from build123d import *

# Parameters (mm, degrees)
F0_R           = 1.6
F1_DEPTH       = 4
F2_W           = 15.6
F2_H           = 14.6
F3_DEPTH       = 5.4
F4_W           = 15.6
F4_H           = 3
F5_DEPTH       = 0.4
F8_D           = 2
F8_DEPTH       = 5
F8_TIP         = 0.600860619
F8_ON_F7_D     = 2
F8_ON_F7_DEPTH = 5
F8_ON_F7_TIP   = 0.600860619
F10_DEPTH      = 25
F12_DEPTH      = 3


with BuildPart() as f1:
    # F0 (on Front) → F1 (new body)
    with BuildSketch(Plane.XZ):
        with BuildLine():
            Line((-7.8, 6.3143593539), (-7.8, 0))
            Line((-7.8, 0), (7.8, 0))
            Line((7.8, 0), (7.8, 6.3143593539))
            ThreePointArc((7.8, 6.3143593539), (5.4, 7.7), (7.8, 9.0856406461))
            Line((7.8, 9.0856406461), (7.8, 20.2))
            Line((7.8, 20.2), (-7.8, 20.2))
            Line((-7.8, 20.2), (-7.8, 9.0856406461))
            ThreePointArc((-7.8, 9.0856406461), (-6.2, 9.0856406461), (-5.4, 7.7))
            ThreePointArc((-5.4, 7.7), (-6.2, 6.3143593539), (-7.8, 6.3143593539))
        make_face()
        with Locations((0, 17.7)):
            Circle(F0_R, mode=Mode.SUBTRACT)
    extrude(amount=F1_DEPTH)

    # F2 (on Front) → F3 (join)
    with BuildSketch(Plane.XZ):
        with Locations((0, -2.7)):
            Rectangle(F2_W, F2_H)
    extrude(amount=-F3_DEPTH)

    # F4 (on face) → F5 (join)
    with BuildSketch(Plane.XZ):
        with Locations((0, -8.5)):
            Rectangle(F4_W, F4_H)
    extrude(amount=F5_DEPTH)

    # F8
    with Locations(Plane.YZ.offset(7.8)):
        with Locations((2.9, -5)):
            Hole(F8_D / 2, depth=F8_DEPTH)
            with Locations((0, 0, -(F8_DEPTH + F8_TIP / 2))):  # 118° drill point
                Cone(0, F8_D / 2, F8_TIP, mode=Mode.SUBTRACT)

    # F8 on F7
    with Locations(Plane(origin=(-7.8, 0, 0), x_dir=(0, -1, 0), z_dir=(-1, 0, 0))):
        with Locations((-2.9, -5)):
            Hole(F8_ON_F7_D / 2, depth=F8_ON_F7_DEPTH)
            with Locations((0, 0, -(F8_ON_F7_DEPTH + F8_ON_F7_TIP / 2))):  # 118° drill point
                Cone(0, F8_ON_F7_D / 2, F8_ON_F7_TIP, mode=Mode.SUBTRACT)

    # F9 (on face) → F10 (cut)
    with BuildSketch(Plane(origin=(0, 0, -10), x_dir=(1, 0, 0), z_dir=(0, 0, -1))):
        Polygon((-6.3, -2.9), (-7.8, -1.4), (-7.8, -4.4), align=None)
        Polygon((7.8, -4.4), (7.8, -1.4), (6.3, -2.9), align=None)
    extrude(amount=-F10_DEPTH, mode=Mode.SUBTRACT)

    # F11 (on face) → F12 (cut, through all)
    with BuildSketch(Plane(origin=(0, 0, -10), x_dir=(1, 0, 0), z_dir=(0, 0, -1))):
        Polygon((-0.25, 0.4), (0, 0.15), (0.25, 0.4), align=None)
    extrude(amount=-F12_DEPTH, mode=Mode.SUBTRACT)


solid = f1.part
Read the model definition and answer for the solid it produces. Units are mm, in the model's axes. A direction names the side the tool comes from. Round coordinates to 2 decimals unless told otherwise and drop trailing zeros. Write each loop counter-clockwise with the first axis right and the second up, starting at its lowest first coordinate (ties: lowest second). Pieces come first, ordered by that corner, then holes. Notation, with made-up numbers: (11.5, 80) - (25.5, 80) arc R24 cw to (25.5, 109) - close; hole circle Ø3 at (47.25, -28). An arc over 180 degrees is marked (long way). One line per question, with ' | ' between items. Start each with the question number.
1. Each of these flat-tipped pins is pushed along its axis until it touches: pin 1 (1.2 mm diameter, centred on y = 2.9, z = -5, fed in from -X); pin 2 (8 mm diameter, centred on x = -3.5, z = 16, fed in from +Y); pin 3 (3 mm diameter, centred on y = 1.5, z = -5.5, fed in from +X); pin 4 (2 mm diameter, centred on x = 2, z = -5, fed in from -Y). Where does it stop, or does it pass through?
2. For a pull along Y with two mould halves and no side action, classify faces 6 (the face through (0, -2, 0)), 7 (the face through (-7, 2.2, -2.8)), 8 (the face through (4, -0.4, -8)) as +Y half, -Y half, draft (parallel to the pull), parting line (faces both ways), or undercut.
3. Find the intervals of material crossed by probe 1 along Z at (x, y) = (-5.9, 2.9); probe 2 along Z at (x, y) = (0, -1.55); probe 3 along Y at (x, z) = (-5.95, -5), in increasing order. Write a range as [from, to].
4. Section B-B (y = -2.5) is taken. Determine the outline of the cut face in (x, z), and give its area (3 significant figures).
5. Section D-D (z = 2.5) is taken. Determine the outline of the cut face in (x, y).
6. Section C-C (x = 2.5) is taken. Determine the outline of the cut face in (y, z), and give its area (3 significant figures).
7. For faces 1 (the face through (0, 0, 13)), 2 (the face through (-4, -0.4, -8)), 3 (the face through (5.4, -2, 7.7)), 4 (the face through (0, 5.4, -3)), 5 (the face through (7.1, 2.1, -2.8)), determine the directions among +Z, -Z, +X, -X, +Y, -Y from which every point of the face is accessible in a straight line to the end or side of a thin tool.
8. Section A-A (x = 7) is taken. Determine the outline of the cut face in (y, z), and give its area (3 significant figures).
Filled in:
1) pin 1: x = -2.56 | pin 2: y = 0 | pin 3: x = 7.8 | pin 4: y = 0
2) face 6: draft | face 7: undercut | face 8: -Y half
3) probe 1: [-10, -6], [-4, 4.6] | probe 2: [0, 16.1], [19.3, 20.2] | probe 3: [0, 1.9], [3.9, 5.4]
4) outline: (-7.8, 0) - (7.8, 0) - (7.8, 6.31) arc R1.6 cw (long way) to (7.8, 9.09) - (7.8, 20.2) - (-7.8, 20.2) - (-7.8, 9.09) arc R1.6 cw (long way) to (-7.8, 6.31) - close; hole circle Ø3.2 at (0, 17.7) | area: 294 mm²
5) outline: (-7.8, -4) - (7.8, -4) - (7.8, 1.4) - (6.3, 2.9) - (7.8, 4.4) - (7.8, 5.4) - (-7.8, 5.4) - (-7.8, 4.4) - (-6.3, 2.9) - (-7.8, 1.4) - close
6) outline: (-4, 0) - (0, 0) - (0, -7) - (-0.4, -7) - (-0.4, -10) - (5.4, -10) - (5.4, 4.6) - (0, 4.6) - (0, 20.2) - (-4, 20.2) - close; hole circle Ø1 at (2.9, -5) | area: 160 mm²
7) face 1: +Z, +X, -X, +Y | face 2: -Z, +X, -X, -Y | face 3: +Y, -Y | face 4: +Z, -Z, +X, -X, +Y | face 5: +Z, -Z, +X
8) outline: (-4, 0) - (0, 0) - (0, -7) - (-0.4, -7) - (-0.4, -10) - (2.2, -10) - (2.2, -5.71) arc R1 cw to (2.2, -4.29) - (2.2, 4.6) - (0, 4.6) - (0, 6.1) - (-4, 6.1) - close; (-4, 9.3) - (0, 9.3) - (0, 20.2) - (-4, 20.2) - close; (3.6, -10) - (5.4, -10) - (5.4, 4.6) - (3.6, 4.6) - (3.6, -4.29) arc R1 cw to (3.6, -5.71) - close | area: 127 mm²
